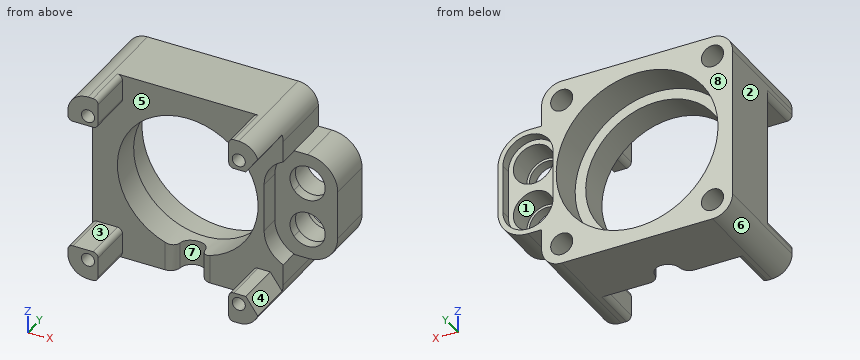
```python
from build123d import *

# Parameters (mm, degrees)
SKETCH1_W                      = 38
SKETCH1_H                      = 38
BOSS_EXTRUDE1_DEPTH            = 22
SKETCH2_R                      = 16.1
CUT_EXTRUDE1_DEPTH             = 7
SKETCH2_3_R                    = 14
CUT_EXTRUDE3_DEPTH             = 35.727510708
FILLET1_R                      = 4
CBORE_FOR_M2_SHCS1_D           = 2.6
CBORE_FOR_M2_SHCS1_CBORE_D     = 4.4
CBORE_FOR_M2_SHCS1_CBORE_DEPTH = 5
CUT_EXTRUDE5_DEPTH             = 9
FILLET2_R                      = 1
CHAMFER1_DEPTH                 = 9
CUT_EXTRUDE6_DEPTH             = 35.727510708
FILLET3_R                      = 2
BOSS_EXTRUDE4_DEPTH            = 9
CUT_EXTRUDE8_DEPTH             = 41.150211222
SKETCH12_R                     = 4
CUT_EXTRUDE9_DEPTH             = 7
SKETCH13_R                     = 6.5
CUT_EXTRUDE11_DEPTH            = 13
CUT_EXTRUDE12_DEPTH            = 2


with BuildPart() as part:
    # Sketch1 → Boss-Extrude1 (new body)
    with BuildSketch(Plane(origin=(0, 0, 0), x_dir=(1, 0, 0), z_dir=(0, 1, 0))):
        Rectangle(SKETCH1_W, SKETCH1_H)
    extrude(amount=BOSS_EXTRUDE1_DEPTH)

    # Sketch2 → Cut-Extrude1 (cut)
    with BuildSketch(Plane(origin=(0, 22, 0), x_dir=(1, 0, 0), z_dir=(0, 1, 0))):
        with Locations(Location((0, 0, 0), (0, 0, 270))):
            Circle(SKETCH2_R)
    extrude(amount=-CUT_EXTRUDE1_DEPTH, mode=Mode.SUBTRACT)

    # Sketch2<3> → Cut-Extrude3 (cut, through all)
    with BuildSketch(Plane(origin=(0, 22, 0), x_dir=(1, 0, 0), z_dir=(0, 1, 0))):
        with Locations(Location((0, 0, 0), (0, 0, 270))):
            Circle(SKETCH2_3_R)
    extrude(amount=-CUT_EXTRUDE3_DEPTH, mode=Mode.SUBTRACT)

    # Fillet1
    fillet1_edges = [part.edges().sort_by_distance(p)[0] for p in [
        (19, 11, 19),
        (-19, 11, 19),
        (-19, 11, -19),
        (19, 11, -19),
    ]]
    fillet(fillet1_edges, radius=FILLET1_R)

    # CBORE for M2 SHCS1 (through all)
    with Locations(Plane(origin=(0, 22, 0), x_dir=(1, 0, 0), z_dir=(0, 1, 0))):
        with Locations((-15, 15), (15, 15), (-15, -15), (15, -15)):
            CounterBoreHole(CBORE_FOR_M2_SHCS1_D / 2, CBORE_FOR_M2_SHCS1_CBORE_D / 2, CBORE_FOR_M2_SHCS1_CBORE_DEPTH)

    # Sketch8 → Cut-Extrude5 (cut)
    with BuildSketch(Plane.XZ):
        Polygon((13, 13), (20, 13), (20, -13), (13, -13), (13, -20), (-13, -20), (-13, -13), (-20, -13), (-20, 13), (-13, 13), (-13, 20), (13, 20), align=None)
    extrude(amount=-CUT_EXTRUDE5_DEPTH, mode=Mode.SUBTRACT)

    # Fillet2
    fillet2_edges = [part.edges().sort_by_distance(p)[0] for p in [
        (13, 4.5, 19),
        (13, 4.5, 13),
        (13, 4.5, -19),
        (13, 4.5, -13),
        (-13, 4.5, -19),
        (-19, 4.5, -13),
        (-13, 4.5, -13),
        (-19, 4.5, 13),
        (-13, 4.5, 19),
        (-13, 4.5, 13),
    ]]
    fillet(fillet2_edges, radius=FILLET2_R)

    # Chamfer1: read off the stored shape, not the designer's step
    # Chamfer1 outline → Chamfer1 (cut)
    with BuildSketch(Plane(origin=(0, 0, 0), x_dir=(1, 0, 0), z_dir=(0, 1, 0))):
        with BuildLine():
            ThreePointArc((19, 15), (18.942394239, 15.676407915), (18.771236167, 16.333333333))
            Line((18.771236167, 16.333333333), (16.414213562, 13))
            Line((16.414213562, 13), (19, 13))
            Line((19, 13), (19, 15))
        make_face()
        with BuildLine():
            Line((19, -15), (19, -13))
            Line((19, -13), (16.414213562, -13))
            Line((16.414213562, -13), (18.771236167, -16.333333333))
            ThreePointArc((18.771236167, -16.333333333), (18.942394239, -15.676407915), (19, -15))
        make_face()
    extrude(amount=CHAMFER1_DEPTH, mode=Mode.SUBTRACT)

    # Sketch10 → Cut-Extrude6 (cut, through all)
    with BuildSketch(Plane.XY):
        with BuildLine():
            Line((2.5, 10.55), (2.5, 0))
            Line((2.5, 0), (-2.5, 0))
            Line((-2.5, 0), (-2.5, 10.55))
            ThreePointArc((-2.5, 10.55), (0, 13.05), (2.5, 10.55))
        make_face()
    extrude(amount=-CUT_EXTRUDE6_DEPTH, mode=Mode.SUBTRACT)

    # Fillet3
    fillet3_edges = [part.edges().sort_by_distance(p)[0] for p in [
        (-2.5, 9, -16.387488657),
        (2.5, 9, -16.387488657),
    ]]
    fillet(fillet3_edges, radius=FILLET3_R)

    # Sketch11 → Boss-Extrude4 (add)
    with BuildSketch(Plane(origin=(0, 22, 0), x_dir=(1, 0, 0), z_dir=(0, 1, 0))):
        with BuildLine():
            Line((19, 7.055118245), (19, 2.589962887))
            ThreePointArc((19, 2.589962887), (22.882033078, 1.529808424), (25.195477121, 4.822540566))
            ThreePointArc((25.195477121, 4.822540566), (22.882033078, 8.115272708), (19, 7.055118245))
        make_face()
        with BuildLine():
            ThreePointArc((19, 7.055118245), (18.195477121, 4.822540566), (19, 2.589962887))
            Line((19, 2.589962887), (19, 7.055118245))
        make_face()
        with BuildLine():
            Line((19, -2.589962887), (19, -7.055118245))
            ThreePointArc((19, -7.055118245), (22.882033078, -8.115272708), (25.195477121, -4.822540566))
            ThreePointArc((25.195477121, -4.822540566), (22.882033078, -1.529808424), (19, -2.589962887))
        make_face()
        with BuildLine():
            ThreePointArc((19, -2.589962887), (18.195477121, -4.822540566), (19, -7.055118245))
            Line((19, -7.055118245), (19, -2.589962887))
        make_face()
        with BuildLine():
            Line((19, -10.822540566), (21.695477121, -10.822540566))
            ThreePointArc((21.695477121, -10.822540566), (25.938117808, -9.065181253), (27.695477121, -4.822540566))
            Line((27.695477121, -4.822540566), (27.695477121, 4.822540566))
            ThreePointArc((27.695477121, 4.822540566), (25.938117808, 9.065181253), (21.695477121, 10.822540566))
            Line((21.695477121, 10.822540566), (19, 10.822540566))
            Line((19, 10.822540566), (19, 7.055118245))
            ThreePointArc((19, 7.055118245), (22.882033078, 8.115272708), (25.195477121, 4.822540566))
            ThreePointArc((25.195477121, 4.822540566), (22.882033078, 1.529808424), (19, 2.589962887))
            Line((19, 2.589962887), (19, -2.589962887))
            ThreePointArc((19, -2.589962887), (22.882033078, -1.529808424), (25.195477121, -4.822540566))
            ThreePointArc((25.195477121, -4.822540566), (22.882033078, -8.115272708), (19, -7.055118245))
            Line((19, -7.055118245), (19, -10.822540566))
        make_face()
    extrude(amount=-BOSS_EXTRUDE4_DEPTH)

    # Sketch11<5> → Cut-Extrude8 (cut, through all)
    with BuildSketch(Plane(origin=(0, 22, 0), x_dir=(1, 0, 0), z_dir=(0, 1, 0))):
        with BuildLine():
            Line((19, 7.055118245), (19, 2.589962887))
            ThreePointArc((19, 2.589962887), (22.882033078, 1.529808424), (25.195477121, 4.822540566))
            ThreePointArc((25.195477121, 4.822540566), (22.882033078, 8.115272708), (19, 7.055118245))
        make_face()
        with BuildLine():
            ThreePointArc((19, 7.055118245), (18.195477121, 4.822540566), (19, 2.589962887))
            Line((19, 2.589962887), (19, 7.055118245))
        make_face()
        with BuildLine():
            Line((19, -2.589962887), (19, -7.055118245))
            ThreePointArc((19, -7.055118245), (22.882033078, -8.115272708), (25.195477121, -4.822540566))
            ThreePointArc((25.195477121, -4.822540566), (22.882033078, -1.529808424), (19, -2.589962887))
        make_face()
        with BuildLine():
            ThreePointArc((19, -2.589962887), (18.195477121, -4.822540566), (19, -7.055118245))
            Line((19, -7.055118245), (19, -2.589962887))
        make_face()
    extrude(amount=-CUT_EXTRUDE8_DEPTH, mode=Mode.SUBTRACT)

    # Sketch12 → Cut-Extrude9 (cut)
    with BuildSketch(Plane(origin=(0, 22, 0), x_dir=(1, 0, 0), z_dir=(0, 1, 0))):
        with Locations(Location((21.695477121, -4.822540566, 0), (0, 0, 270))):
            Circle(SKETCH12_R)
        with Locations(Location((21.695477121, 4.822540566, 0), (0, 0, 270))):
            Circle(SKETCH12_R)
    extrude(amount=-CUT_EXTRUDE9_DEPTH, mode=Mode.SUBTRACT)

    # Sketch13 → Cut-Extrude11 (cut)
    with BuildSketch(Plane.XZ):
        with Locations((21.695477121, -4.822540566)):
            Circle(SKETCH13_R)
        with Locations((21.695477121, 4.822540566)):
            Circle(SKETCH13_R)
        with BuildLine():
            ThreePointArc((17.337369448, 0), (15.755035223, 2.184141418), (15.195477121, 4.822540566))
            Line((15.195477121, 4.822540566), (15.195477121, -4.822540566))
            ThreePointArc((15.195477121, -4.822540566), (15.755035223, -2.184141418), (17.337369448, 0))
        make_face()
    extrude(amount=-CUT_EXTRUDE11_DEPTH, mode=Mode.SUBTRACT)

    # Sketch15 → Cut-Extrude12 (cut)
    with BuildSketch(Plane(origin=(0, 22, 0), x_dir=(1, 0, 0), z_dir=(0, 1, 0))):
        with BuildLine():
            Line((16.695477121, -4.822540566), (16.695477121, 4.822540566))
            ThreePointArc((16.695477121, 4.822540566), (21.695477121, 9.822540566), (26.695477121, 4.822540566))
            Line((26.695477121, 4.822540566), (26.695477121, -4.822540566))
            ThreePointArc((26.695477121, -4.822540566), (21.695477121, -9.822540566), (16.695477121, -4.822540566))
        make_face()
    extrude(amount=-CUT_EXTRUDE12_DEPTH, mode=Mode.SUBTRACT)


solid = part.part
```
Geometry check sheet. Reference: the model listing, model coordinates, mm. Face numbers are marked on the shaded views. A direction names the side the tool comes from. Give positions to 0.01 mm unless a question says otherwise; leave off trailing zeros. Write each loop counter-clockwise with the first axis right and the second up, starting at its lowest first coordinate (ties: lowest second). Pieces come first, ordered by that corner, then holes.
1) Release check for a two-part mould opening along X. For the marked faces 6, 7 and 8 record: pulls with the +X half, pulls with the -X half, needs draft (parallel to the pull), parting line crosses it, or undercut.
2) Section check C-C, the plane x = 0. Record the boundary of the cut face in (y, z), and give its area (4 significant figures).
3) Access from +Z, -Z, +X, -X, +Y, -Y to the whole of each face (thin tool, end or side, straight path). Record for the marked faces 1, 2, 3, 4 and 5.
4) Section check D-D, the plane y = 18. Record the boundary of the cut face in (x, z), and give its area (3 significant figures).
5) Gauge pin test, flat ends, axial feed: pin 1 (1.2 mm diameter, centred on y = 11, z = -1.5, fed in from +X); pin 2 (2.5 mm diameter, centred on x = -15, z = 15, fed in from -Y); pin 3 (2 mm diameter, centred on y = 13, z = 12, fed in from +X); pin 4 (1.2 mm diameter, centred on x = -17, y = 5.5, fed in from -Z). Record the tip position at first contact, or that the pin passes through.
6) Material ranges on L1, parallel to Z at x = 15, y = 5.5; L2, parallel to Z at x = 15, y = 13; L3, parallel to X at y = 10, z = 16, recorded low to high.
7) Section check B-B, the plane z = 0. Record the boundary of the cut face in (x, y).
8) Section check A-A, the plane y = 8. State how many separate pieces and enclosed holes the cut face has, and give its area (3 significant figures).
Computed:
1. face 6: pulls with the -X half
1. face 7: undercut
1. face 8: needs draft
2. outline: (9, 14) - (15, 14) - (15, 16.1) - (22, 16.1) - (22, 19) - (9, 19) - close; (13.05, -19) - (22, -19) - (22, -16.1) - (15, -16.1) - (15, -14) - (13.05, -14) - close
2. area: 80.35 mm2
3. face 1: +Y
3. face 2: +Z, -Z, -X, +Y, -Y
3. face 3: +X, -X, -Y
3. face 4: +X, -Y
3. face 5: -Y
4. outline: (-19, -15) arc R4 ccw to (-15, -19) - (15, -19) arc R4 ccw to (19, -15) - (19, -10.82) - (21.7, -10.82) arc R6 ccw to (27.7, -4.82) - (27.7, 4.82) arc R6 ccw to (21.7, 10.82) - (19, 10.82) - (19, 15) arc R4 ccw to (15, 19) - (-15, 19) arc R4 ccw to (-19, 15) - close; hole circle Ø4.4 at (-15, -15); hole circle Ø4.4 at (-15, 15); hole circle Ø32.2 at (0, 0); hole circle Ø4.4 at (15, -15); hole circle Ø4.4 at (15, 15); hole circle Ø8 at (21.7, -4.82); hole circle Ø8 at (21.7, 4.82)
4. area: 627 mm2
5. pin 1: stops at x = 15.2
5. pin 2: passes through
5. pin 3: stops at x = 19
5. pin 4: stops at z = -18.75
6. L1: z = -19 to -16.3, -13.7 to -13, 13 to 13.7, 16.3 to 19
6. L2: z = -19 to -16.3, -13.7 to 13.7, 16.3 to 19
6. L3: x = -18.87 to -15.83, -14.17 to 14.17, 15.83 to 18.87
7. outline: (-19, 9) - (-14, 9) - (-14, 15) - (-16.1, 15) - (-16.1, 22) - (-19, 22) - close; (14, 9) - (15.2, 9) - (15.2, 13) - (27.7, 13) - (27.7, 22) - (26.7, 22) - (26.7, 20) - (16.7, 20) - (16.7, 22) - (16.1, 22) - (16.1, 15) - (14, 15) - close
8. separate pieces: 4
8. enclosed holes: 4
8. area: 97.7 mm2
